from build123d import *

# Parameters (mm, degrees)
EXTRUDE_1_DEPTH     = 4.04
EXTRUDE_START       = 3
EXTRUDE_2_DEPTH     = 3
EXTRUDE_3_DEPTH     = 6
CUT_EXTRUDE_1_DEPTH = 69.95015268178993
CUT_EXTRUDE_2_DEPTH = 5
DRAFT_1_ANGLE       = 60.000000000000234
CUT_EXTRUDE_3_REACH = 69.351
SKETCH_6_R          = 2.000000000000003
SKETCH_7_R          = 2.002237129098131
CUT_EXTRUDE_4_DEPTH = 5
RIB_1_REACH         = 68.835
SKETCH_8_WALL_W     = 141.6697430182401
SKETCH_8_WALL_H     = 2
FILLET_1_R          = 10
FILLET_2_R          = 10


with BuildPart() as part:
    # 草图1 → 凸台-拉伸1 (new body)
    with BuildSketch(Plane.XY):
        with BuildLine():
            Line((2.711712708194342, 12.202320033019019), (59.53806556534447, 5.964171430093859))
            ThreePointArc((59.53806556534447, 5.964171430093859), (64.81417632321985, -0.9084264437888516), (57.72286495852592, -5.886704197633859))
            ThreePointArc((57.72286495852592, -5.886704197633859), (36.58461274967972, -5.515977162880489), (16.63, -12.5))
            Line((16.63, -12.5), (0, -12.5))
            ThreePointArc((0, -12.5), (-12.425357146028794, 1.364001390626533), (2.711712708194342, 12.202320033019019))
        make_face()
    extrude(amount=EXTRUDE_1_DEPTH)

    # 草图2 → 凸台-拉伸2 (add)
    with BuildSketch(Plane(origin=(0, 0, 0), x_dir=(-1, 0, 0), z_dir=(0, 0, -1)).offset(EXTRUDE_START)):
        with BuildLine():
            Line((-16.629999999999995, -12.500000000000004), (2.3e-15, -12.5))
            ThreePointArc((2.3e-15, -12.5), (12.425357146028796, 1.3640013906265342), (-2.711712708194334, 12.202320033019022))
            Line((-2.711712708194334, 12.202320033019022), (-59.53806556534447, 5.964171430093854))
            ThreePointArc((-59.53806556534447, 5.964171430093854), (-64.81417632321985, -0.9084264437888536), (-57.72286495852591, -5.886704197633859))
            ThreePointArc((-57.72286495852591, -5.886704197633859), (-36.584612749679714, -5.515977162880482), (-16.629999999999995, -12.500000000000004))
        make_face()
    extrude(amount=-EXTRUDE_2_DEPTH)

    # 草图3 → 凸台-拉伸3 (add)
    with BuildSketch(Plane.XY.offset(4.04)):
        with BuildLine():
            Line((31.302864958525912, 9.063708323856956), (59.53806556534447, 5.964171430093859))
            ThreePointArc((59.53806556534447, 5.964171430093859), (64.81417632321985, -0.9084264437888548), (57.72286495852591, -5.886704197633853))
            ThreePointArc((57.72286495852591, -5.886704197633853), (44.47245462008017, -4.776317380993831), (31.302864958525912, -6.611594244587196))
            Line((31.302864958525912, -6.611594244587196), (31.302864958525912, 9.063708323856956))
        make_face()
    extrude(amount=EXTRUDE_3_DEPTH)

    # 草图4 → 切除-拉伸1 (cut, through all)
    with BuildSketch(Plane(origin=(1.3558563540964497, 12.351160016509516, 0), x_dir=(0.9940285716823101, -0.10912011125006546, 0), z_dir=(0.10912011125006545, 0.99402857168231, 0))):
        with BuildLine():
            Line((45.761727224680776, -5.039999999999999), (58.53172722468078, -5.04))
            Line((58.53172722468078, -5.04), (58.53172722468078, 0.96))
            Line((58.53172722468078, 0.96), (39.06172722468078, 0.9599999999999976))
            ThreePointArc((39.06172722468078, 0.9599999999999976), (38.05523868595962, 0.06182278930871615), (38.83352399440517, -1.040000000000001))
            Line((38.83352399440517, -1.040000000000001), (45.761727224680776, -5.039999999999999))
        make_face()
    extrude(amount=-CUT_EXTRUDE_1_DEPTH, mode=Mode.SUBTRACT)

    # 草图5 → 切除-拉伸2 (cut)
    with BuildSketch(Plane.XY.offset(4.04)):
        with BuildLine():
            Line((3.6299942497491204, 4.727481587079438), (17.823503151893238, 2.570486685801488))
            ThreePointArc((17.823503151893238, 2.570486685801488), (20.032864958525913, 0), (17.823503151893238, -2.5704866858014865))
            Line((17.823503151893238, -2.5704866858014865), (3.62999424974912, -4.72748158707944))
            ThreePointArc((3.62999424974912, -4.72748158707944), (-7.084043052340996, 7.8e-16), (3.6299942497491204, 4.727481587079438))
        make_face()
    extrude(amount=-CUT_EXTRUDE_2_DEPTH, mode=Mode.SUBTRACT)

    # 拔模1
    draft_1_faces = [part.faces().sort_by_distance(p)[0] for p in [
        (31.302864958525912, 1.226057039634884, 7.04),
    ]]
    draft(draft_1_faces, Plane(origin=(58.88334489784406, 0, 4.04), x_dir=(1, 0, 0), z_dir=(0, 0, 1)), DRAFT_1_ANGLE)

    # 切除-拉伸3: up to this face of the body (flat: up to its plane)
    cut_extrude_3_end = Plane(part.part.faces().sort_by_distance((20.783576678, 0.227997431, -3))[0])
    # 草图6 → 切除-拉伸3 (cut, up to the picked face)
    with BuildSketch(Plane.XY.offset(10.040000000000001), mode=Mode.PRIVATE) as cut_extrude_3_sk1:
        with Locations((58.88334489784406, 0)):
            Circle(SKETCH_6_R)
    cut_extrude_3_tool1 = split(extrude(cut_extrude_3_sk1.sketch, amount=-CUT_EXTRUDE_3_REACH, mode=Mode.PRIVATE), bisect_by=cut_extrude_3_end, keep=Keep.BOTH, mode=Mode.PRIVATE)
    add(cut_extrude_3_tool1.solids().sort_by(Axis((58.883345, 0, 10.04), (0, 0, -1)))[0], mode=Mode.SUBTRACT)

    # 草图7 → 切除-拉伸4 (cut)
    with BuildSketch(Plane.XY.offset(-0.96)):
        Circle(SKETCH_7_R)
    extrude(amount=-CUT_EXTRUDE_4_DEPTH, mode=Mode.SUBTRACT)

    # 草图8 wall → 筋1 (add, up to next)
    with BuildSketch(Plane(origin=(50.454320705, 0, 2.04), x_dir=(0, 0, -1), z_dir=(-1, 0, 0)), mode=Mode.PRIVATE) as rib_1_sk1:
        Rectangle(SKETCH_8_WALL_W, SKETCH_8_WALL_H)
    rib_1_tool1 = extrude(rib_1_sk1.sketch, amount=RIB_1_REACH, mode=Mode.PRIVATE) - part.part
    add(rib_1_tool1.solids().sort_by_distance((50.454320705, 0, 2.04))[0])

    # 圆角1
    fillet_1_edges = [part.edges().sort_by_distance(p)[0] for p in [
        (16.629999999999992, -12.5, 0.52),
    ]]
    fillet(fillet_1_edges, radius=FILLET_1_R)

    # 圆角2
    fillet_2_edges = [part.edges().sort_by_distance(p)[0] for p in [
        (31.302864958525912, 1.2260570396348758, 4.04),
        (41.69516980393928, 1.5029507858131876, 10.04),
        (3.629994249749121, 4.727481587079438, 1.54),
        (3.62999424974912, -4.72748158707944, 1.54),
    ]]
    fillet(fillet_2_edges, radius=FILLET_2_R)


solid = part.part
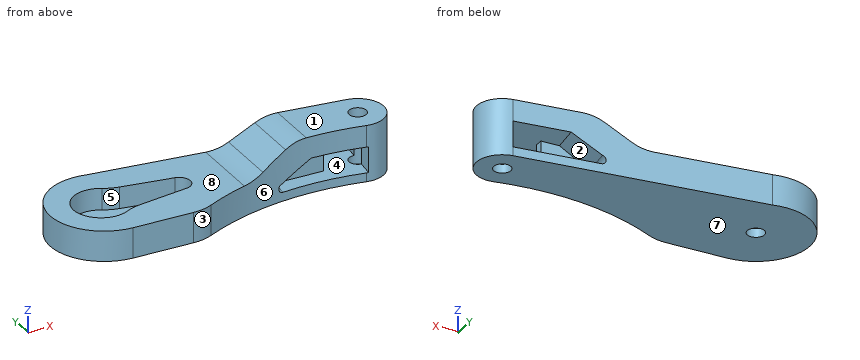
Could you check a few things on this model? Use its own coordinates, in mm. Face numbers are marked on the shaded views. A direction names the side the tool comes from. Give positions to 0.01 mm unless a question says otherwise; leave off trailing zeros. Order: outer loops, then holes, each group sorted by start corner. A loop starts at its lowest first (then second) coordinate and runs counter-clockwise, first axis right, second up. Notation, with made-up numbers: (-26, 7) - (25, 7) arc R5 ccw to (25, 16) - close; hole circle Ø5 at (-37.75, 17.5). An arc over 180 degrees is marked (long way). One line per item, written item: value. Start each with the question number.
1. For the marked faces 4, 5, 6, 7 and 8, which set-ups out of +Z, -Z, +X, -X, +Y, -Y let a thin tool reach every point of the face, with its end or its side?
2. Imagine slicing it at A-A on y = 0. List the corners of the cut face in (x, z) for me, plus the area to 3 significant figures.
3. Imagine slicing it at B-B on x = 52. List the corners of the cut face in (y, z) for me, plus the area to 3 significant figures.
4. Thinking about a two-plate mould opening in X: for the marked faces 1, 2 and 3, which applies, +X half, -X half, draft (parallel to the pull), parting line (faces both ways), or undercut?
5. For P1, Ø5, axis at y = 5.5, z = -0.5, coming from the +X side; P2, Ø1.8, axis at x = 46.5, z = 0.5, coming from the -Y side; P3, Ø12, axis at x = 23, y = -3.5, coming from the +Z side, each with a flat end and sliding along its axis, tell me the tip position at first contact or that it passes through.
6. Imagine slicing it at C-C on z = -2. List the corners of the cut face in (x, y) for me.
7. Imagine slicing it at D-D on x = 4.5. List the corners of the cut face in (y, z) for me, plus the area to 3 significant figures.
8. If I drill on probe 1 along Y at (x, z) = (0, -1.4); probe 2 along Y at (x, z) = (18, 2.25); probe 3 along Z at (x, y) = (14, 6.75), over which ranges is the centre line in solid material (lowest first)?
Values:
1. face 4: none
1. face 5: +Z
1. face 6: +Z, -Z, -Y
1. face 7: -Z, +X, -X, +Y, -Y
1. face 8: +Z, -X, +Y, -Y
2. outline: (-12.5, -3) - (-2, -3) - (-2, -0.96) - (-7.08, -0.96) - (-7.08, 4.04) - (-12.5, 4.04) - close; (2, -3) - (56.88, -3) - (56.88, -0.96) - (50.45, -0.96) - (50.45, 5.04) - (56.88, 5.04) - (56.88, 10.04) - (44.37, 10.04) arc R10 ccw to (39.37, 8.7) - (33.62, 5.38) arc R10 cw to (28.62, 4.04) - (20.03, 4.04) - (20.03, -0.96) - (2, -0.96) - close; (60.88, -3) - (64.88, -3) - (64.88, 10.04) - (60.88, 10.04) - close
2. area: 481 mm²
3. outline: (-5.04, -3) - (6.79, -3) - (6.79, -0.96) - (-5.04, -0.96) - close; (-5.04, 5.04) - (6.79, 5.04) - (6.79, 10.04) - (-5.04, 10.04) - close
3. area: 83.3 mm²
4. face 1: draft
4. face 2: undercut
4. face 3: +X half
5. P1: x = 64.08
5. P2: y = -1
5. P3: z = 4.05
6. outline: (0, -12.5) - (14.11, -12.5) arc R10 ccw to (18.68, -11.39) arc R60 cw to (57.72, -5.89) arc R6 ccw (long way) to (59.54, 5.96) - (2.71, 12.2) arc R12.5 ccw (long way) to start; hole circle Ø4 at (0, 0); hole circle Ø4 at (58.88, 0)
7. outline: (-12.5, -3) - (12.01, -3) - (12.01, 4.04) - (4.7, 4.04) - (4.7, -0.96) - (-4.7, -0.96) - (-4.7, 4.04) - (-12.5, 4.04) - close
7. area: 126 mm²
8. probe 1: -12.5 to -2, 2 to 12.5
8. probe 2: -11.71 to -2.54, 2.54 to 10.52
8. probe 3: -3 to 4.04
